from build123d import *

# Parameters (mm, degrees)
F0_W     = 1000
F0_H     = 1000
F1_DEPTH = 25
F2_SIZE  = 10
F3_SIZE  = 10


with BuildPart() as f1:
    # F0 (on Top) → F1 (new body)
    with BuildSketch(Plane.XY):
        with BuildLine():
            Line((0, 943.124099), (0, -56.875901))
            ThreePointArc((0, -56.875901), (500, 443.124099), (0, 943.124099))
        make_face()
        with Locations((-500, 443.124099)):
            Rectangle(F0_W, F0_H)
        with BuildLine():
            ThreePointArc((-1000, 943.124099), (-1500, 443.124099), (-1000, -56.875901))
            Line((-1000, -56.875901), (-1000, 943.124099))
        make_face()
    extrude(amount=-F1_DEPTH)

    # F2
    f2_edges = [f1.edges().sort_by_distance(p)[0] for p in [
        (500, 443.124099, -25),
        (-500, 943.124099, -25),
        (-1500, 443.124099, -25),
        (-500, -56.875901, -25),
    ]]
    chamfer(f2_edges, length=F2_SIZE)

    # F3
    f3_edges = [f1.edges().sort_by_distance(p)[0] for p in [
        (-500, 943.124099, 0),
    ]]
    chamfer(f3_edges, length=F3_SIZE)


solid = f1.part
Input: part model. Units: mm. Frame: model coordinates. Coordinates: 2 decimals unless noted, no trailing zeros. Loops run counter-clockwise (first coordinate to the right, second up) from the corner with the lowest first, then second, coordinate; pieces in that order, holes last.
(1) Material intervals for probe 1 along Y at (x, z) = (-1100, -14.25); probe 2 along X at (y, z) = (677, -18.75); probe 3 along Y at (x, z) = (-1203, -12), sorted ascending.
(2) Section A-A on z = -20.5. Return the cut outline in (x, y), then the cut area to 3 significant figures.
(3) First-contact query: pin 1 Ø2 at (y, z) = (169.5, -18.5) entering from -X; pin 2 Ø6 at (x, z) = (-384, -20.5) entering from -Y; pin 3 Ø6 at (y, z) = (149, -3.5) entering from -X. Flat tips, straight axial feed; report the tip coordinate or a pass-through.
Data:
1. probe 1: y = -46.77 to 933.02
1. probe 2: x = -1437.68 to 437.68
1. probe 3: y = -13.81 to 900.06
2. outline: (-1000, -51.38) - (0, -51.38) arc R494.5 ccw to (0, 937.62) - (-1000, 937.62) arc R494.5 ccw to start
2. area: 1,760,000 mm2
3. pin 1: stops at x = -1415.66
3. pin 2: stops at y = -54.38
3. pin 3: stops at x = -1400.61
